from build123d import *

# Parameters (mm, degrees)
SKETCH1_R           = 2.35
BOSS_EXTRUDE1_DEPTH = 10.5
SKETCH2_R           = 4.75
BOSS_EXTRUDE2_DEPTH = 6.9
SKETCH3_R           = 7.95
BOSS_EXTRUDE3_DEPTH = 1.64
SKETCH4_R           = 7.715
BOSS_EXTRUDE4_DEPTH = 1.8


# Read off the part's stored shape, not the designer's step: Loft1
with BuildPart() as part:
    # Sketch1 → Boss-Extrude1 (new body)
    with BuildSketch(Plane(origin=(0, 0, 0), x_dir=(1, 0, 0), z_dir=(0, 1, 0))):
        with Locations(Location((0, 0, 0), (0, 0, 90))):
            Circle(SKETCH1_R)
    extrude(amount=BOSS_EXTRUDE1_DEPTH)

    # Sketch2 → Boss-Extrude2 (add)
    with BuildSketch(Plane.XZ):
        with Locations(Location((0, 0, 0), (0, 0, 90))):
            Circle(SKETCH2_R)
    extrude(amount=BOSS_EXTRUDE2_DEPTH)

    # Sketch3 → Boss-Extrude3 (add)
    with BuildSketch(Plane.XZ.offset(6.9)):
        with Locations(Location((0, 0, 0), (0, 0, 270))):
            Circle(SKETCH3_R)
    extrude(amount=BOSS_EXTRUDE3_DEPTH)

    # Sketch4 → Boss-Extrude4 (add)
    with BuildSketch(Plane.XZ.offset(8.54)):
        with Locations(Location((0, 0, 0), (0, 0, 270))):
            Circle(SKETCH4_R)
    extrude(amount=BOSS_EXTRUDE4_DEPTH)

    # Loft1 outline → Loft1 (revolve)
    with BuildSketch(Plane.XY):
        Polygon((0, -10.34), (0, -91.19), (7.35, -91.19), (9, -10.34), align=None)
    revolve(axis=Axis((0, 0, 0), (0, 1, 0)))


solid = part.part
CAD build for the part. Positions are in the model's coordinates, mm. A direction names the side the tool comes from. Coordinates: 2 decimals unless noted, no trailing zeros. Loops run counter-clockwise (first coordinate to the right, second up) from the corner with the lowest first, then second, coordinate; pieces in that order, holes last. Notation, with made-up numbers: (-26.5, -34.75) - (2.5, -34.75) arc R11 cw to (2.5, -15.75) - close; hole circle Ø7 at (40.25, -38.75). An arc over 180 degrees is marked (long way). Write item = value, one per line. Start each with the question number.
Q1. Cut at C-C, the plane y = -81.5. List the corners of the cut face in (x, z), then the cut area to 3 significant figures.
Q2. Flat gauge pins, fed straight in: pin 1 Ø10 at (y, z) = (-70, -2.5) entering from -X; pin 2 Ø6 at (y, z) = (-32.5, -3) entering from -X; pin 3 Ø2 at (y, z) = (-80, 5.5) entering from +X. Where does each tip first touch, or does it go through?
Q3. Cut at B-B, the plane z = 0. List the corners of the cut face in (x, y) (3 decimals), then the cut area to 3 significant figures.
Q4. Cut at D-D, the plane y = -39. List the corners of the cut face in (x, z), then the cut area to 3 significant figures.
Q5. Pull direction Y, two halves, no side cores. Call faces 1 (the cylindrical face through (-4.837, -7.709, 6.309)), 2 (the flat face through (2, 0, 2)), 3 (the flat face through (0, -91.19, 0)), 4 (the cylindrical face through (-6.845, -9.427, -3.56)): pulls with the +Y half, pulls with the -Y half, needs draft (parallel to the pull), parting line crosses it, or undercut.
Q6. Which spindle directions (+Z, -Z, +X, -X, +Y, -Y) get a long thin tool onto all of the face, cutting with end or side? Do faces 5 (the cylindrical face through (-0.71, 5.18, -2.24)), 6 (the conical face through (-1.066, -50.199, -8.117)), 7 (the flat face through (0, 10.5, 0)), 8 (the flat face through (7, -10.34, -4)). Say none if no direction does.
Q7. Drill centre lines: L1, parallel to Y at x = -3.25, z = -5.5; L2, parallel to X at y = -30.5, z = -3.25; L3, parallel to Y at x = 4, z = 2.5. Where is each one in solid material? Low to high.
Q8. Cut at A-A, the plane x = 0. List the corners of the cut face in (y, z) (3 decimals), then the cut area to 3 significant figures.
Computed:
q1.outline = circle Ø15.1 at (0, 0)
q1.area = 179 mm²
q2.pin_1 = -7.87
q2.pin_2 = -8.57
q2.pin_3 = 6.1
q3.outline = (-9, -10.34) - (-7.35, -91.19) - (7.35, -91.19) - (9, -10.34) - (7.715, -10.34) - (7.715, -8.54) - (7.95, -8.54) - (7.95, -6.9) - (4.75, -6.9) - (4.75, 0) - (2.35, 0) - (2.35, 10.5) - (-2.35, 10.5) - (-2.35, 0) - (-4.75, 0) - (-4.75, -6.9) - (-7.95, -6.9) - (-7.95, -8.54) - (-7.715, -8.54) - (-7.715, -10.34) - close
q3.area = 1,490 mm²
q4.outline = circle Ø16.83 at (0, 0)
q4.area = 222 mm²
q5.face_1 = needs draft
q5.face_2 = pulls with the +Y half
q5.face_3 = pulls with the -Y half
q5.face_4 = undercut
q6.face_5 = +Y
q6.face_6 = -Y
q6.face_7 = +Z, -Z, +X, -X, +Y
q6.face_8 = none
q7.L1 = -91.19 to -6.9
q7.L2 = -7.95 to 7.95
q7.L3 = -91.19 to 0
q8.outline = (-91.19, -7.35) - (-10.34, -9) - (-10.34, -7.715) - (-8.54, -7.715) - (-8.54, -7.95) - (-6.9, -7.95) - (-6.9, -4.75) - (0, -4.75) - (0, -2.35) - (10.5, -2.35) - (10.5, 2.35) - (0, 2.35) - (0, 4.75) - (-6.9, 4.75) - (-6.9, 7.95) - (-8.54, 7.95) - (-8.54, 7.715) - (-10.34, 7.715) - (-10.34, 9) - (-91.19, 7.35) - close
q8.area = 1,490 mm²
